Print and shaded views of the part. All mm, measured from the part's lowest x, y and z. A direction names the side the tool comes from. Coordinates: 2 decimals unless noted, no trailing zeros. Loops run counter-clockwise (first coordinate to the right, second up) from the corner with the lowest first, then second, coordinate; pieces in that order, holes last.
1) Pin check, flat tips, straight feed: pin 1 Ø10 at (x, z) = (24, 22.5) entering from +Y; pin 2 Ø10 at (x, y) = (36, 95) entering from -Z; pin 3 Ø1 at (x, y) = (15, 54) entering from +Z. Stop position of each tip, or through.
2) Wall check: line 1 along Y through (x, z) = (81, 105.5); line 2 along X through (y, z) = (16.5, 81); line 3 along Z through (x, y) = (39, 91.5) (1 decimal). Give the ranges that are in metal, low to high.
3) Saw through at A-A, the plane x = 30. Write the cut outline in (y, z) (1 decimal), and give its area (3 significant figures).
4) Saw through at C-C, the plane z = 24. Write the cut outline in (x, y), and give its area (3 significant figures).
5) Saw through at D-D, the plane z = 80. Write the cut outline in (x, y).
6) Which spindle directions (+Z, -Z, +X, -X, +Y, -Y) get a long thin tool onto all of the face, cutting with end or side? Do the marked faces 1 and 2. Say none if no direction does.
7) Saw through at B-B, the plane y = 38. Write the cut outline in (x, z).
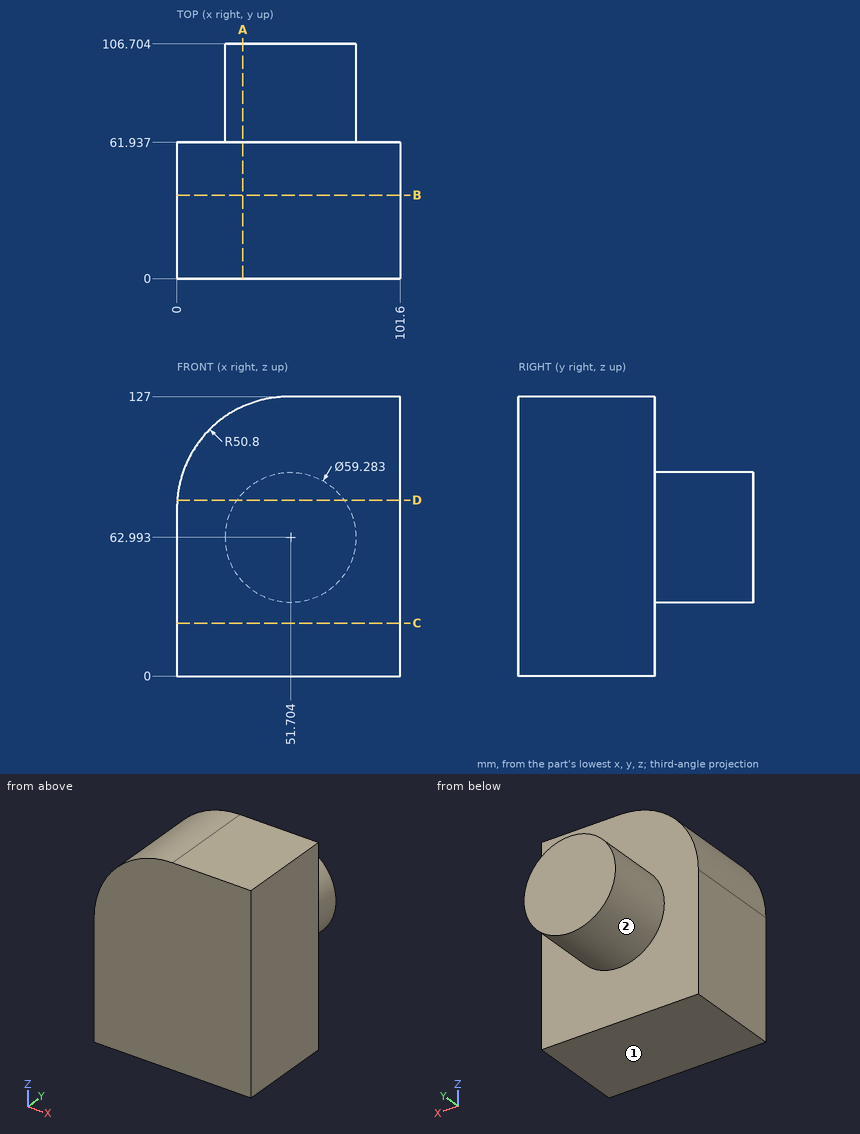
Data:
1. pin 1: stops at y = 61.94
1. pin 2: stops at z = 35.35
1. pin 3: stops at z = 112.73
2. line 1: y = 0 to 61.94
2. line 2: x = 0.23 to 101.6
2. line 3: z = 36.2 to 89.8
3. outline: (0, 0) - (61.9, 0) - (61.9, 42.8) - (106.7, 42.8) - (106.7, 83.2) - (61.9, 83.2) - (61.9, 122.5) - (0, 122.5) - close
3. area: 9,400 mm2
4. outline: (0, 0) - (101.6, 0) - (101.6, 61.94) - (0, 61.94) - close
4. area: 6,290 mm2
5. outline: (0.14, 0) - (101.6, 0) - (101.6, 61.94) - (75.98, 61.94) - (75.98, 106.7) - (27.43, 106.7) - (27.43, 61.94) - (0.14, 61.94) - close
6. face 1: -Z, +X, -X, +Y, -Y
6. face 2: +Y
7. outline: (0, 0) - (101.6, 0) - (101.6, 127) - (50.8, 127) arc R50.8 ccw to (0, 76.2) - close
